Drawing for the job (mm, zero at the part's lowest x, y, z). Round coordinates to 2 decimals unless told otherwise and drop trailing zeros. Order: outer loops, then holes, each group sorted by start corner. A loop starts at its lowest first (then second) coordinate and runs counter-clockwise, first axis right, second up. Notation, with made-up numbers: (61.25, -7) - (81.25, -7) arc R15 cw to (81.25, 8) - close; hole circle Ø3 at (77.25, -29.75). An arc over 180 degrees is marked (long way). Put each result on its own line as item: value. Start each with the question number.
Item 1: Saw through at D-D on x = 62. List the corners of the cut face in (y, z).
Item 2: Saw through at A-A on x = 110.2. List the corners of the cut face in (y, z).
Item 3: Saw through at B-B on z = 0.8. State how many separate pieces and enclosed holes the cut face has, plus the area to 3 significant figures.
Item 4: Saw through at C-C on y = 3. List the corners of the cut face in (x, z), plus the area to 3 significant figures.
Item 5: Probe probe 1 along Y at (x, z) = (2.5, 1.5); probe 2 along X at (y, z) = (11.5, 2.35); probe 3 along X at (y, z) = (33, 0.5). List the from-to ranges inside material, lowest first.
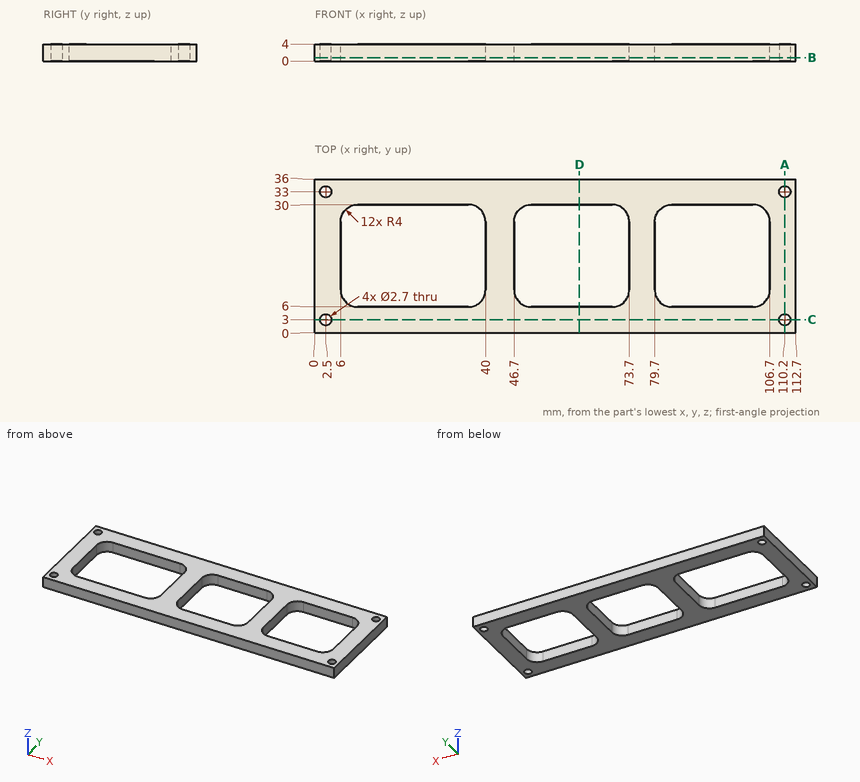
Results found:
1. outline: (0, 0) - (6, 0) - (6, 4) - (0, 4) - close; (30, 0) - (36, 0) - (36, 4) - (30, 4) - close
2. outline: (0, 0) - (1.65, 0) - (1.65, 4) - (0, 4) - close; (4.35, 0) - (31.65, 0) - (31.65, 4) - (4.35, 4) - close; (34.35, 0) - (36, 0) - (36, 4) - (34.35, 4) - close
3. separate pieces: 1
3. enclosed holes: 7
3. area: 1,960 mm²
4. outline: (0, 0) - (1.15, 0) - (1.15, 4) - (0, 4) - close; (3.85, 0) - (108.85, 0) - (108.85, 4) - (3.85, 4) - close; (111.55, 0) - (112.7, 0) - (112.7, 4) - (111.55, 4) - close
4. area: 429 mm²
5. probe 1: y = 0 to 1.65, 4.35 to 31.65, 34.35 to 36
5. probe 2: x = 0 to 6, 40 to 46.7, 73.7 to 79.7, 106.7 to 112.7
5. probe 3: x = 0 to 1.15, 3.85 to 108.85, 111.55 to 112.7
